Part model, mm, in its own coordinate system. Coordinates: 2 decimals unless noted, no trailing zeros. Loops run counter-clockwise (first coordinate to the right, second up) from the corner with the lowest first, then second, coordinate; pieces in that order, holes last. Notation, with made-up numbers: (57, 13) - (77, 13) arc R21 cw to (77, 50) - close; hole circle Ø1 at (47.25, -33.75). An arc over 180 degrees is marked (long way). Answer as CSV lines item,"result".
from build123d import *

# Parameters (mm, degrees)
SKETCH1_R           = 22.5
BOSS_EXTRUDE1_DEPTH = 24
CHAMFER1_SIZE       = 1
SKETCH2_R           = 1.5
CUT_EXTRUDE1_DEPTH  = 40.855990767


with BuildPart() as part:
    # Sketch1 → Boss-Extrude1 (new body)
    with BuildSketch(Plane(origin=(0, 0, 0), x_dir=(1, 0, 0), z_dir=(0, 1, 0))):
        with Locations(Location((0, 0, 0), (0, 0, 270))):
            Circle(SKETCH1_R)
    extrude(amount=BOSS_EXTRUDE1_DEPTH)

    # Chamfer1
    chamfer1_edges = [part.edges().sort_by_distance(p)[0] for p in [
        (0, 0, -22.5),
        (0, 24, -22.5),
    ]]
    chamfer(chamfer1_edges, length=CHAMFER1_SIZE)

    # Sketch2 → Cut-Extrude1 (cut, through all)
    with BuildSketch(Plane(origin=(0, 24, 0), x_dir=(1, 0, 0), z_dir=(0, 1, 0))):
        with Locations(Location((14.5, 0, 0), (0, 0, 270))):
            Circle(SKETCH2_R)
    extrude(amount=-CUT_EXTRUDE1_DEPTH, mode=Mode.SUBTRACT)


solid = part.part
Q1. Flat gauge pins, fed straight in: pin 1 (1 mm diameter, centred on x = -12.5, y = 6.5, fed in from -Z); pin 2 (5 mm diameter, centred on y = 7.5, z = -2.5, fed in from +X); pin 3 (1.5 mm diameter, centred on x = -8, y = 6, fed in from +Z); pin 4 (1.5 mm diameter, centred on x = -17, z = -8.5, fed in from -Y). Where does each tip first touch, or does it go through?
Results:
pin 1,"stops at z = -19.03"
pin 2,"stops at x = 22.5"
pin 3,"stops at z = 21.3"
pin 4,"stops at y = 0"
Q2. Wall check: L1, parallel to X at y = 12, z = 0; L2, parallel to X at y = 20.75, z = 0.5; L3, parallel to X at y = 14.5, z = -18. Give the ranges that are in metal, low to high.
Results:
L1,"x = -22.5 to 13, 16 to 22.5"
L2,"x = -22.49 to 13.09, 15.91 to 22.49"
L3,"x = -13.5 to 13.5"
Q3. Two-plate mould, pull along Z, no slides. Class faces 1 (the face through (-8.618, 11.846, 20.784)), 2 (the face through (14.95, 12.17, 1.43)), 3 (the face through (0, 24, 0)): released by +Z, released by -Z, zero draft, split by the parting line, or undercut.
Results:
face 1,"split by the parting line"
face 2,"undercut"
face 3,"zero draft"
Q4. Saw through at A-A (z = 0). Give the cut face in (x, y), then the cut area to 3 significant figures.
Results:
outline,"(-22.5, 1) - (-21.5, 0) - (13, 0) - (13, 24) - (-21.5, 24) - (-22.5, 23) - close; (16, 0) - (21.5, 0) - (22.5, 1) - (22.5, 23) - (21.5, 24) - (16, 24) - close"
area,"1,010 mm^2"
Q5. Saw through at B-B (y = 15.5). Give the cut face in (x, z), then the cut area to 3 significant figures.
Results:
outline,"circle Ø45 at (0, 0); hole circle Ø3 at (14.5, 0)"
area,"1,580 mm^2"
